Build history of the part. All positions in model axes, mm. A direction names the side the tool comes from. Give positions to 0.01 mm unless a question says otherwise; leave off trailing zeros. Order: outer loops, then holes, each group sorted by start corner. A loop starts at its lowest first (then second) coordinate and runs counter-clockwise, first axis right, second up. Notation, with made-up numbers: (68.25, 66) - (107.25, 66) arc R26 ccw to (107.25, 105) - close; hole circle Ø1 at (2.25, -27). An arc over 180 degrees is marked (long way). Use a Markdown table: item, result. Add a question column.
(1) Mould opens along Z. For faces 1 (the face through (75, 1, 76.2)), 2 (the face through (69.747, 33.084, -0.121)), 3 (the face through (75, 37.85, -18)) say: +Z half, -Z half, draft (parallel to the pull), parting line (faces both ways), or undercut.
(2) Slice it at D-D (z = 47). Write the cut outline in (x, y), then the cut area to 3 significant figures.
(3) Slice it at A-A (x = 75). Write the cut outline in (y, z), then the cut area to 3 significant figures.
(4) Which spindle directions (+Z, -Z, +X, -X, +Y, -Y) get a long thin tool onto all of the face, cutting with end or side? Do faces 4 (the face through (75, -4, -69.9)), 5 (the face through (0, 31, 0)). Say none if no direction does.
(5) Wall check: line 1 (Z direction, x = 148, y = 0) (3 decimals); line 2 (Z direction, x = 75, y = 31); line 3 (Z direction, x = 27.5, y = -18). Give the ranges that are in metal, low to high.
(6) Slice it at C-C (x = 100.5). Write the cut outline in (y, z), then the cut area to 3 significant figures.
(7) Slice it at B-B (y = -17). Write the cut outline in (x, z).
(8) Flat gauge pins, fed straight in: pin 1 (5 mm diameter, centred on x = 97, z = 7.5, fed in from -Y); pin 2 (1.5 mm diameter, centred on y = 32.85, z = 73.025, fed in from +X); pin 3 (3.5 mm diameter, centred on x = 67, z = -8, fed in from +Y); pin 4 (1.5 mm diameter, centred on y = 0, z = 73.025, fed in from -X). Where does each tip first touch, or does it go through?
from build123d import *

# Parameters (mm, degrees)
BOSS_EXTRUDE1_DEPTH        = 151.4
F_12_0_12_DIAMETER_HOLE1_D = 8
F_10_0_10_DIAMETER_HOLE1_D = 8
M3_TAPPED_HOLE1_D          = 2.5
M3_TAPPED_HOLE1_DEPTH      = 7.5
M3_TAPPED_HOLE1_TIP        = 0.751075774
M5_CLEARANCE_HOLE1_D       = 5.5
SKETCH19_R                 = 3
CUT_EXTRUDE3_DEPTH         = 186.631058824


with BuildPart() as part:
    # Sketch1 → Boss-Extrude1 (new body)
    with BuildSketch(Plane(origin=(0, 0, 0), x_dir=(0, 0, -1), z_dir=(1, 0, 0))):
        with BuildLine():
            Line((-69.9, -36.85), (-69.9, 27.45))
            ThreePointArc((-69.9, 27.45), (-69.607106781, 28.157106781), (-68.9, 28.45))
            Line((-68.9, 28.45), (68.9, 28.45))
            ThreePointArc((68.9, 28.45), (69.607106781, 28.157106781), (69.9, 27.45))
            Line((69.9, 27.45), (69.9, -36.85))
            ThreePointArc((69.9, -36.85), (70.192893219, -37.557106781), (70.9, -37.85))
            Line((70.9, -37.85), (75.2, -37.85))
            ThreePointArc((75.2, -37.85), (75.907106781, -37.557106781), (76.2, -36.85))
            Line((76.2, -36.85), (76.2, 36.85))
            ThreePointArc((76.2, 36.85), (75.907106781, 37.557106781), (75.2, 37.85))
            Line((75.2, 37.85), (-75.2, 37.85))
            ThreePointArc((-75.2, 37.85), (-75.907106781, 37.557106781), (-76.2, 36.85))
            Line((-76.2, 36.85), (-76.2, -36.85))
            ThreePointArc((-76.2, -36.85), (-75.907106781, -37.557106781), (-75.2, -37.85))
            Line((-75.2, -37.85), (-70.9, -37.85))
            ThreePointArc((-70.9, -37.85), (-70.192893219, -37.557106781), (-69.9, -36.85))
        make_face()
    extrude(amount=BOSS_EXTRUDE1_DEPTH)

    # Ø12.0 (12) Diameter Hole1 (through all)
    with Locations(Plane(origin=(0, 37.85, 0), x_dir=(1, 0, 0), z_dir=(0, 1, 0))):
        with Locations((75, 0)):
            Hole(F_12_0_12_DIAMETER_HOLE1_D / 2)

    # Ø10.0 (10) Diameter Hole1 (through all)
    with Locations(Plane(origin=(0, 37.85, 0), x_dir=(1, 0, 0), z_dir=(0, 1, 0))):
        with Locations((75, -12.5), (75, 0), (75, 12.5)):
            Hole(F_10_0_10_DIAMETER_HOLE1_D / 2)

    # M3 Tapped Hole1
    with Locations(Plane(origin=(151.4, 0, 0), x_dir=(0, 0, -1), z_dir=(1, 0, 0))):
        with Locations((-73.025, 0), (-73.025, 32.85), (0, 33.575019096), (73.025, 0), (73.025, 32.85)):
            Hole(M3_TAPPED_HOLE1_D / 2, depth=M3_TAPPED_HOLE1_DEPTH)
            with Locations((0, 0, -(M3_TAPPED_HOLE1_DEPTH + M3_TAPPED_HOLE1_TIP / 2))):  # 118° drill point
                Cone(0, M3_TAPPED_HOLE1_D / 2, M3_TAPPED_HOLE1_TIP, mode=Mode.SUBTRACT)

    # M5 Clearance Hole1 (through all)
    with Locations(Plane(origin=(0, 37.85, 0), x_dir=(1, 0, 0), z_dir=(0, 1, 0))):
        with Locations((83, 0), (67, 0)):
            Hole(M5_CLEARANCE_HOLE1_D / 2)

    # Sketch19 → Cut-Extrude3 (cut, through all)
    with BuildSketch(Plane(origin=(0, 37.85, 0), x_dir=(1, 0, 0), z_dir=(0, 1, 0))):
        with Locations(Location((67, 8, 0), (0, 0, 270))):
            Circle(SKETCH19_R)
        with Locations(Location((83, 8, 0), (0, 0, 270))):
            Circle(SKETCH19_R)
        with Locations(Location((83, -8, 0), (0, 0, 270))):
            Circle(SKETCH19_R)
        with Locations(Location((67, -8, 0), (0, 0, 270))):
            Circle(SKETCH19_R)
    extrude(amount=-CUT_EXTRUDE3_DEPTH, mode=Mode.SUBTRACT)


solid = part.part
Solution:
| question | item | result |
|---|---|---|
| 1 | face 1 | +Z half |
| 1 | face 2 | undercut |
| 1 | face 3 | draft |
| 2 | outline | (0, 28.45) - (151.4, 28.45) - (151.4, 37.85) - (0, 37.85) - close |
| 2 | area | 1,420 mm2 |
| 3 | outline | (-37.85, -75.2) arc R1 ccw to (-36.85, -76.2) - (36.85, -76.2) arc R1 ccw to (37.85, -75.2) - (37.85, -16.5) - (28.45, -16.5) - (28.45, -68.9) arc R1 cw to (27.45, -69.9) - (-36.85, -69.9) arc R1 ccw to (-37.85, -70.9) - close; (-37.85, 70.9) arc R1 ccw to (-36.85, 69.9) - (27.45, 69.9) arc R1 cw to (28.45, 68.9) - (28.45, 16.5) - (37.85, 16.5) - (37.85, 75.2) arc R1 ccw to (36.85, 76.2) - (-36.85, 76.2) arc R1 ccw to (-37.85, 75.2) - close; (28.45, -8.5) - (37.85, -8.5) - (37.85, -4) - (28.45, -4) - close; (28.45, 4) - (37.85, 4) - (37.85, 8.5) - (28.45, 8.5) - close |
| 3 | area | 2,040 mm2 |
| 4 | face 4 | +X, -X, -Y |
| 4 | face 5 | +Z, -Z, -X, +Y, -Y |
| 5 | line 1 | -76.2 to -74.275, -71.775 to -69.9, 69.9 to 71.775, 74.275 to 76.2 |
| 5 | line 2 | -76.2 to -16.5, -8.5 to -4, 4 to 8.5, 16.5 to 76.2 |
| 5 | line 3 | -76.2 to -69.9, 69.9 to 76.2 |
| 6 | outline | (-37.85, -75.2) arc R1 ccw to (-36.85, -76.2) - (36.85, -76.2) arc R1 ccw to (37.85, -75.2) - (37.85, 75.2) arc R1 ccw to (36.85, 76.2) - (-36.85, 76.2) arc R1 ccw to (-37.85, 75.2) - (-37.85, 70.9) arc R1 ccw to (-36.85, 69.9) - (27.45, 69.9) arc R1 cw to (28.45, 68.9) - (28.45, -68.9) arc R1 cw to (27.45, -69.9) - (-36.85, -69.9) arc R1 ccw to (-37.85, -70.9) - close |
| 6 | area | 2,270 mm2 |
| 7 | outline | (0, -76.2) - (151.4, -76.2) - (151.4, -69.9) - (0, -69.9) - close; (0, 69.9) - (151.4, 69.9) - (151.4, 76.2) - (0, 76.2) - close |
| 8 | pin 1 | y = 28.45 |
| 8 | pin 2 | x = 143.6 |
| 8 | pin 3 | through |
| 8 | pin 4 | x = 0 |
